```python
from build123d import *

# Parameters (mm, degrees)
BOSS_EXTRUDE1_DEPTH = 1.5
SKETCH3_R           = 1.5
SKETCH3_R_2         = 1.55
CUT_EXTRUDE1_DEPTH  = 1.5
SKETCH10_W          = 5
SKETCH10_H          = 6
SKETCH10_R          = 0.85
CUT_EXTRUDE5_DEPTH  = 167.982783544
SKETCH8_R           = 0.85
CUT_EXTRUDE4_DEPTH  = 10


with BuildPart() as part:
    # Sketch1 → Boss-Extrude1 (new body)
    with BuildSketch(Plane.XY):
        Polygon((140, 0), (0, 0), (0, -91), (140, -91), (140, -70.5), (120, -70.5), (120, -20.5), (140, -20.5), align=None)
    extrude(amount=BOSS_EXTRUDE1_DEPTH)

    # Sketch3 → Cut-Extrude1 (cut)
    with BuildSketch(Plane.XY.offset(1.5)):
        with Locations((18, -40.5)):
            Circle(SKETCH3_R)
        with Locations((96, -58)):
            Circle(SKETCH3_R_2)
        with BuildLine():
            Line((97.55, -19.439908336), (97.55, -36.560091664))
            ThreePointArc((97.55, -36.560091664), (96, -38.110091664), (94.45, -36.560091664))
            Line((94.45, -36.560091664), (94.45, -19.439908336))
            ThreePointArc((94.45, -19.439908336), (96, -17.889908336), (97.55, -19.439908336))
        make_face()
    extrude(amount=-CUT_EXTRUDE1_DEPTH, mode=Mode.SUBTRACT)

    # Sketch10 → Cut-Extrude5 (cut, through all)
    with BuildSketch(Plane.XY.offset(1.5)):
        with Locations((2.5, -10.5)):
            Rectangle(SKETCH10_W, SKETCH10_H)
        with Locations((2.5, -80.5)):
            Rectangle(SKETCH10_W, SKETCH10_H)
        with Locations((137.5, -10.5)):
            Rectangle(SKETCH10_W, SKETCH10_H)
        with Locations((137.5, -80.5)):
            Rectangle(SKETCH10_W, SKETCH10_H)
        with Locations((8.45, -10.5)):
            Circle(SKETCH10_R)
        with Locations((8.45, -80.5)):
            Circle(SKETCH10_R)
        with Locations((131.55, -10.5)):
            Circle(SKETCH10_R)
        with Locations((131.55, -80.5)):
            Circle(SKETCH10_R)
    extrude(amount=-CUT_EXTRUDE5_DEPTH, mode=Mode.SUBTRACT)

    # Sketch8 → Cut-Extrude4 (cut)
    with BuildSketch(Plane.ZY):
        with Locations((0.75, -38.75)):
            Circle(SKETCH8_R)
        with Locations((0.75, 31.25)):
            Circle(SKETCH8_R)
    extrude(amount=-CUT_EXTRUDE4_DEPTH, mode=Mode.SUBTRACT)


solid = part.part
```
Input: part model. Units: mm. Frame: model coordinates. Give positions to 0.01 mm unless a question says otherwise; leave off trailing zeros. Order: outer loops, then holes, each group sorted by start corner. A loop starts at its lowest first (then second) coordinate and runs counter-clockwise, first axis right, second up. Notation, with made-up numbers: (68, 57) - (87, 57) arc R13 ccw to (87, 66) - close; hole circle Ø5 at (28, 25.25). An arc over 180 degrees is marked (long way). One line per item, written item: value.
1. Line query: probe 1 along Y at (x, z) = (131.55, 0.4); probe 2 along Y at (x, z) = (8.45, 0.8); probe 3 along X at (y, z) = (-19.5, 1.1). Output: solid intervals per line, ascending.
Determined:
probe 1: -91 to -81.35, -79.65 to -70.5, -20.5 to -11.35, -9.65 to 0
probe 2: -91 to -81.35, -79.65 to -39.6, -37.9 to -11.35, -9.65 to 0
probe 3: 0 to 94.45, 97.55 to 140
2. Cut plane A-A, the plane y = -58. Output: boundary loops of the cut face in (x, z), and give its area (3 significant figures).
Determined:
outline: (0, 0) - (94.45, 0) - (94.45, 1.5) - (0, 1.5) - close; (97.55, 0) - (120, 0) - (120, 1.5) - (97.55, 1.5) - close
area: 175 mm2
3. Cut plane B-B, the plane y = -47. Output: boundary loops of the cut face in (x, z).
Determined:
outline: (0, 0) - (120, 0) - (120, 1.5) - (0, 1.5) - close
4. Cut plane C-C, the plane z = 0.25. Give the number of separate pieces and of enclosed holes in the cut face, and give its area (3 significant figures).
Determined:
separate pieces: 1
enclosed holes: 7
area: 11,500 mm2
5. Pin query (flat end, axial travel): pin 1 Ø0.8 at (y, z) = (-30.5, 1) entering from +X; pin 2 Ø0.8 at (y, z) = (-38.5, 0.5) entering from -X. Return the tip coordinate at first contact, or that it passes through.
Determined:
pin 1: x = 120
pin 2: x = 10
6. Draft query along X for faces 1 (the face through (16.8, -41.4, 0.8)), 2 (the face through (69, -45, 0)). Return one class per face: released by +X, released by -X, zero draft, split by the parting line, or undercut.
Determined:
face 1: undercut
face 2: zero draft
